Can you work these out from the model? Positions are in its coordinate system, mm. Face numbers are marked on the shaded views. A direction names the side the tool comes from. Give positions to 0.01 mm unless a question says otherwise; leave off trailing zeros. Order: outer loops, then holes, each group sorted by start corner. A loop starts at its lowest first (then second) coordinate and runs counter-clockwise, first axis right, second up. Notation, with made-up numbers: (64.25, -40) -> (113.25, -40) arc R28 cw to (113.25, -20) -> close; hole circle Ø9 at (-35.75, 21.25). An arc over 180 degrees is marked (long way). Answer as CSV lines item,"result".
```python
from build123d import *
from build123d.topology import SkipClean

# Parameters (mm, degrees)
BOSS_EXTRUDE1_DEPTH     = 5
BOSS_EXTRUDE2_DEPTH     = 43
CUT_EXTRUDE1_DEPTH      = 99.344878968
CUT_EXTRUDE1_DEPTH_BACK = 99.344878968
SKETCH4_R               = 2.25
CUT_EXTRUDE2_DEPTH      = 14
SKETCH6_R               = 3.75
CUT_EXTRUDE3_DEPTH      = 14
SKETCH7_R               = 2.25
CUT_EXTRUDE4_DEPTH      = 50
CUT_EXTRUDE5_DEPTH      = 28
EXTRUDE_THIN1_DEPTH     = 43
CHAMFER1_SIZE           = 5
CHAMFER2_START          = 4.9999999
CHAMFER2_DEPTH          = 43.0000001
CHAMFER3_SIZE           = 10
CHAMFER3_SIZE_2         = 7.855445392
EXTRUDE_THIN2_REACH     = 99.948


with BuildPart() as part:
    # Sketch1 → Boss-Extrude1 (new body)
    with BuildSketch(Plane.XY):
        with BuildLine():
            Line((0, 21), (31.588461174, 21))
            Line((31.588461174, 21), (50.172213659, 35.135394674))
            ThreePointArc((50.172213659, 35.135394674), (72.920555239, 32.042625706), (69.827786272, 9.294284126))
            Line((69.827786272, 9.294284126), (30, -21))
            Line((30, -21), (0, -21))
            ThreePointArc((0, -21), (-14.491376746, -15.198684154), (-20.976176963, -1))
            Line((-20.976176963, -1), (-7.685213074, -1))
            ThreePointArc((-7.685213074, -1), (7.75, 0), (-7.685213074, 1))
            Line((-7.685213074, 1), (-20.976176963, 1))
            ThreePointArc((-20.976176963, 1), (-14.491376746, 15.198684154), (0, 21))
        make_face()
        with BuildLine():
            Line((27.437787439, 0.273900145), (29.82554698, 2.090106184))
            ThreePointArc((29.82554698, 2.090106184), (32.978521164, 1.661441058), (32.549856038, -1.491533127))
            Line((32.549856038, -1.491533127), (30.162096497, -3.307739166))
            ThreePointArc((30.162096497, -3.307739166), (27.009122313, -2.87907404), (27.437787439, 0.273900145))
        make_face(mode=Mode.SUBTRACT)
        with BuildLine():
            Line((62.556034265, 21.332122764), (60.168274724, 19.515916725))
            ThreePointArc((60.168274724, 19.515916725), (57.01530054, 19.944581851), (57.443965666, 23.097556036))
            Line((57.443965666, 23.097556036), (59.831725206, 24.913762075))
            ThreePointArc((59.831725206, 24.913762075), (62.984699391, 24.485096949), (62.556034265, 21.332122764))
        make_face(mode=Mode.SUBTRACT)
    extrude(amount=BOSS_EXTRUDE1_DEPTH)

    # Sketch2 → Boss-Extrude2 (add)
    with SkipClean():  # the faces are left unmerged after this step: merging them gives an invalid solid
        with BuildSketch(Plane.XY.offset(5)):
            with BuildLine():
                Line((-7.685213074, -1), (-20.976176963, -1))
                ThreePointArc((-20.976176963, -1), (-14.491376746, -15.198684154), (0, -21))
                ThreePointArc((0, -21), (21, 0), (0, 21))
                ThreePointArc((0, 21), (-14.491376746, 15.198684154), (-20.976176963, 1))
                Line((-20.976176963, 1), (-7.685213074, 1))
                ThreePointArc((-7.685213074, 1), (7.75, 0), (-7.685213074, -1))
            make_face()
        extrude(amount=BOSS_EXTRUDE2_DEPTH)
    add(part.part.scale(1), mode=Mode.REPLACE)  # the faces are merged on a copy

    # Sketch4 → Cut-Extrude1 (cut, two sides: drawn at the far end of the back side and taken through both)
    with SkipClean():  # the faces are left unmerged after this step: merging them gives an invalid solid
        with BuildSketch(Plane(origin=(0, -1, 0), x_dir=(1, 0, 0), z_dir=(0, 1, 0)).offset(-CUT_EXTRUDE1_DEPTH_BACK)):
            with Locations(Location((-14.330695019, -24, 0), (0, 0, 180))):
                Circle(SKETCH4_R)
        extrude(amount=CUT_EXTRUDE1_DEPTH + CUT_EXTRUDE1_DEPTH_BACK, mode=Mode.SUBTRACT)

    # Sketch5 → Cut-Extrude2 (cut)
    with SkipClean():  # the faces are left unmerged after this step: merging them gives an invalid solid
        with BuildSketch(Plane.XZ.offset(21)):
            Polygon((-12.834085604, 19.936730349), (-10.063495571, 23.264466947), (-11.560104986, 27.327736598), (-15.827304434, 28.063269651), (-18.597894467, 24.735533053), (-17.101285052, 20.672263402), align=None)
        extrude(amount=-CUT_EXTRUDE2_DEPTH, mode=Mode.SUBTRACT)

    # Sketch6 → Cut-Extrude3 (cut)
    with SkipClean():  # the faces are left unmerged after this step: merging them gives an invalid solid
        with BuildSketch(Plane(origin=(0, 21, 0), x_dir=(1, 0, 0), z_dir=(0, 1, 0))):
            with Locations(Location((-14.330695019, -24, 0), (0, 0, 270))):
                Circle(SKETCH6_R)
        extrude(amount=-CUT_EXTRUDE3_DEPTH, mode=Mode.SUBTRACT)

    # Sketch7 → Cut-Extrude4 (cut)
    with SkipClean():  # the faces are left unmerged after this step: merging them gives an invalid solid
        with BuildSketch(Plane(origin=(0, 0, 0), x_dir=(-1, 0, 0), z_dir=(0, 0, -1))):
            with Locations((0, 14.375)):
                Circle(SKETCH7_R)
            with Locations((0, -14.375)):
                Circle(SKETCH7_R)
        extrude(amount=-CUT_EXTRUDE4_DEPTH, mode=Mode.SUBTRACT)

    # Sketch8 → Cut-Extrude5 (cut)
    with SkipClean():  # the faces are left unmerged after this step: merging them gives an invalid solid
        with BuildSketch(Plane.XY.offset(48)):
            Polygon((4.156921938, 14.375), (2.078460969, 17.975), (-2.078460969, 17.975), (-4.156921938, 14.375), (-2.078460969, 10.775), (2.078460969, 10.775), align=None)
            Polygon((4.156921938, -14.375), (2.078460969, -10.775), (-2.078460969, -10.775), (-4.156921938, -14.375), (-2.078460969, -17.975), (2.078460969, -17.975), align=None)
        extrude(amount=-CUT_EXTRUDE5_DEPTH, mode=Mode.SUBTRACT)

    # Sketch9 → Extrude-Thin1 (add)
    with SkipClean():  # the faces are left unmerged after this step: merging them gives an invalid solid
        with BuildSketch(Plane.XY.offset(5)):
            with BuildLine():
                Line((0, 21), (31.588461174, 21))
                Line((31.588461174, 21), (50.172213659, 35.135394674))
                ThreePointArc((50.172213659, 35.135394674), (72.920555239, 32.042625706), (69.827786272, 9.294284126))
                Line((69.827786272, 9.294284126), (30, -21))
                Line((30, -21), (0, -21))
                Line((0, -21), (0, -18))
                Line((0, -18), (28.988704289, -18))
                Line((28.988704289, -18), (68.011580233, 11.682043667))
                ThreePointArc((68.011580233, 11.682043667), (70.532795698, 30.226419667), (51.988419698, 32.747635133))
                Line((51.988419698, 32.747635133), (32.599756885, 18))
                Line((32.599756885, 18), (0, 18))
                Line((0, 18), (0, 21))
            make_face()
        extrude(amount=EXTRUDE_THIN1_DEPTH)

    # Chamfer1
    chamfer1_edges = [part.edges().sort_by_distance(p)[0] for p in [
        (21, 0, 5),
        (19.902679058, -18, 5),
        (21.708205356, 18, 5),
        (42.294088292, 25.373817566, 5),
        (70.532795698, 30.226419667, 5),
        (48.500142261, -3.158978166, 5),
    ]]
    chamfer(chamfer1_edges, length=CHAMFER1_SIZE)

    # Chamfer2: read off the stored shape, not the designer's step
    # Chamfer2 outline → Chamfer2 (add)
    with SkipClean():  # the faces are left unmerged after this step: merging them gives an invalid solid
        with BuildSketch(Plane.XY.offset(CHAMFER2_START)):
            with BuildLine():
                Line((10.816653826, -18), (15.091675551, -18))
                Line((15.091675551, -18), (17.124404275, -12.155442329))
                ThreePointArc((17.124404275, -12.155442329), (14.272890231, -15.404045068), (10.816653826, -18))
            make_face()
            with BuildLine():
                ThreePointArc((10.816653826, 18), (14.272890231, 15.404045068), (17.124404275, 12.155442329))
                Line((17.124404275, 12.155442329), (15.091675551, 18))
                Line((15.091675551, 18), (10.816653826, 18))
            make_face()
        extrude(amount=CHAMFER2_DEPTH)

    # Chamfer3
    # the kernel refuses this chamfer: 10, 7.855445392 mm, written as the material it adds along each edge
    with BuildSketch(Plane(origin=(15.091675551, -18, -15.71682988), x_dir=(0.32849742893027223, 0.9445048645646038, 0), z_dir=(0, 0, 1))) as chamfer3_piece_1_section:
        Polygon((CHAMFER3_SIZE, 0), (CHAMFER3_SIZE_2 * 0.328497428916, -CHAMFER3_SIZE_2 * 0.944504864523), (0, 0), align=None)
    chamfer3_piece_1 = extrude(amount=63.71682988, mode=Mode.PRIVATE)
    chamfer3_piece_1 = split(chamfer3_piece_1, bisect_by=Plane(origin=(15.091675551, -5.14158506, -2.85841494), z_dir=(0, 0.7071067811865476, 0.7071067811865476)), keep=Keep.TOP, mode=Mode.PRIVATE)
    add(chamfer3_piece_1)
    with BuildSketch(Plane(origin=(15.091675551, 18, -15.71682988), x_dir=(0.32849742893027223, -0.9445048645646039, 0), z_dir=(0, 0, 1))) as chamfer3_piece_2_section:
        Polygon((CHAMFER3_SIZE, 0), (CHAMFER3_SIZE_2 * 0.328497428916, CHAMFER3_SIZE_2 * 0.944504864523), (0, 0), align=None)
    chamfer3_piece_2 = extrude(amount=63.71682988, mode=Mode.PRIVATE)
    chamfer3_piece_2 = split(chamfer3_piece_2, bisect_by=Plane(origin=(15.091675551, 5.14158506, -2.85841494), z_dir=(0, -0.7071067811865476, 0.7071067811865476)), keep=Keep.TOP, mode=Mode.PRIVATE)
    add(chamfer3_piece_2)

    # Extrude-Thin2: up to this face of the body (flat: up to its plane)
    extrude_thin2_end = Plane(part.part.faces().sort_by_distance((44.470080552, 10.533508587, 5))[0])
    # Sketch10 → Extrude-Thin2 (add, up to the picked face)
    with BuildSketch(Plane.XY.offset(48), mode=Mode.PRIVATE) as extrude_thin2_sk1:
        Polygon((33.519574493, 22.468866363), (53.175147106, -3.372244184), (55.562906646, -1.556038145), (35.907334034, 24.285072402), align=None)
    extrude_thin2_tool1 = split(extrude(extrude_thin2_sk1.sketch, amount=-EXTRUDE_THIN2_REACH, mode=Mode.PRIVATE), bisect_by=extrude_thin2_end, keep=Keep.BOTH, mode=Mode.PRIVATE)
    add(extrude_thin2_tool1.solids().sort_by(Axis((44.541241, 10.456414, 48), (0, 0, -1)))[0])


solid = part.part
```
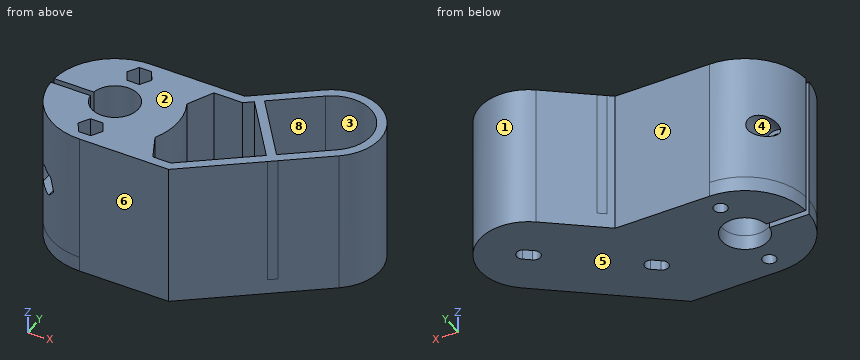
Item 1: For pin 1 (6 mm diameter, centred on y = -9.5, z = 27, fed in from -X); pin 2 (4 mm diameter, centred on x = 0, y = -14.375, fed in from +Z); pin 3 (3.5 mm diameter, centred on x = 0, y = 13.5, fed in from +Z); pin 4 (2 mm diameter, centred on x = -13.5, z = 25.5, fed in from +Y), each with a flat end and sliding along its axis, tell me the tip position at first contact or that it passes through.
Numbers:
pin 1,"stops at x = -19.97"
pin 2,"passes through"
pin 3,"stops at z = 20"
pin 4,"stops at y = 7"
Item 2: Imagine slicing it at B-B, the plane x = 39.5. Please give me the cut outline in (y, z).
Numbers:
outline,"(-13.77, 0) -> (27.02, 0) -> (27.02, 48) -> (23.25, 48) -> (23.25, 10) -> (19.56, 7.07) -> (19.56, 48) -> (14.61, 48) -> (14.61, 5) -> (-3.72, 5) -> (-10, 10) -> (-10, 48) -> (-13.77, 48) -> close"
Item 3: We'd pull the mould along X, two halves only. Please class the marked faces 1, 2 and 3: released by +X, released by -X, zero draft, split by the parting line, or undercut.
Numbers:
face 1,"split by the parting line"
face 2,"zero draft"
face 3,"undercut"
Item 4: Please list where these lines run through material, in increasing order: line 1 along X through (y, z) = (9, 17.5); line 2 along X through (y, z) = (-15, 31); line 3 along X through (y, z) = (5.85, 24).
Numbers:
line 1,"x = -18.97 to 18.97, 43.76 to 47.53, 64.49 to 69.44"
line 2,"x = -14.7 to -3.8, 3.8 to 21.5, 32.93 to 37.89"
line 3,"x = -20.17 to -16.58, -12.08 to -5.08, 5.08 to 20.17, 46.16 to 49.93, 60.34 to 65.3"
Item 5: Imagine slicing it at A-A, the plane z = 39. Give the number of separate pieces and of enclosed holes in the cut face, then the cut area to 3 significant figures.
Numbers:
separate pieces,"1"
enclosed holes,"4"
area,"1,750 mm²"
Item 6: For the marked faces 4, 5, 6, 7 and 8, which set-ups out of +Z, -Z, +X, -X, +Y, -Y let a thin tool reach every point of the face, with its end or its side?
Numbers:
face 4,"+Y"
face 5,"-Z, +X, -X, +Y, -Y"
face 6,"+Z, -Z, +X, -X, -Y"
face 7,"+Z, -Z, -X, +Y"
face 8,"+Z"
